```python
from build123d import *

# Parameters (mm, degrees)
SKETCH1_R           = 4.7
SKETCH1_R_2         = 2.5
BOSS_EXTRUDE1_DEPTH = 2.5
SKETCH2_R           = 4.7
BOSS_EXTRUDE2_DEPTH = 4.5
SKETCH3_R           = 1
CUT_EXTRUDE1_DEPTH  = 4.5
SKETCH6_W           = 6
SKETCH6_H           = 6
BOSS_EXTRUDE3_DEPTH = 8.31
SKETCH7_W           = 6
SKETCH7_H           = 6
BOSS_EXTRUDE4_DEPTH = 2
FILLET1_R           = 1
SKETCH8_R           = 1.75
CUT_EXTRUDE2_DEPTH  = 1.5
BOSS_EXTRUDE5_DEPTH = 0.5


with BuildPart() as part:
    # Sketch1 → Boss-Extrude1 (new body)
    with BuildSketch(Plane(origin=(0, 0, 0), x_dir=(1, 0, 0), z_dir=(0, 1, 0))):
        with Locations(Location((0, 0, 0), (0, 0, 270))):
            Circle(SKETCH1_R)
        with Locations(Location((0, 0, 0), (0, 0, 270))):
            Circle(SKETCH1_R_2, mode=Mode.SUBTRACT)
    extrude(amount=BOSS_EXTRUDE1_DEPTH)

    # Sketch2 → Boss-Extrude2 (add)
    with BuildSketch(Plane(origin=(0, 2.5, 0), x_dir=(1, 0, 0), z_dir=(0, 1, 0))):
        with Locations(Location((0, 0, 0), (0, 0, 270))):
            Circle(SKETCH2_R)
    extrude(amount=BOSS_EXTRUDE2_DEPTH)

    # Sketch3 → Cut-Extrude1 (cut)
    with BuildSketch(Plane(origin=(0, 7, 0), x_dir=(1, 0, 0), z_dir=(0, 1, 0))):
        with Locations(Location((0, 0, 0), (0, 0, 270))):
            Circle(SKETCH3_R)
    extrude(amount=-CUT_EXTRUDE1_DEPTH, mode=Mode.SUBTRACT)



with BuildPart() as body_2:
    # Sketch6 → Boss-Extrude3 (new body)
    with BuildSketch(Plane(origin=(4.7, 0, 0), x_dir=(0, 0, -1), z_dir=(1, 0, 0))):
        with Locations((0, 3.5)):
            Rectangle(SKETCH6_W, SKETCH6_H)
    extrude(amount=BOSS_EXTRUDE3_DEPTH)


with BuildPart() as part_1:
    add(part.part)

    add(body_2.part)  # Boss-Extrude4 merges body 2
    # Sketch7 → Boss-Extrude4 (add)
    with BuildSketch(Plane.ZY.offset(-4.7)):
        with Locations((0, 3.5)):
            Rectangle(SKETCH7_W, SKETCH7_H)
    extrude(amount=BOSS_EXTRUDE4_DEPTH)

    # Fillet1
    fillet1_edges = [part_1.edges().sort_by_distance(p)[0] for p in [
        (13.01, 3.5, -3),
        (13.01, 3.5, 3),
    ]]
    fillet(fillet1_edges, radius=FILLET1_R)

    # Sketch8 → Cut-Extrude2 (cut)
    with BuildSketch(Plane(origin=(13.01, 0, 0), x_dir=(0, 0, -1), z_dir=(1, 0, 0))):
        with Locations((0, 3.5)):
            Circle(SKETCH8_R)
    extrude(amount=-CUT_EXTRUDE2_DEPTH, mode=Mode.SUBTRACT)

    # Sketch9 → Boss-Extrude5 (add)
    with BuildSketch(Plane(origin=(0, 6.5, 0), x_dir=(1, 0, 0), z_dir=(0, 1, 0))):
        with BuildLine():
            Line((13.01, -2), (13.01, 2))
            ThreePointArc((13.01, 2), (12.717106781, 2.707106781), (12.01, 3))
            Line((12.01, 3), (3.618010503, 3))
            ThreePointArc((3.618010503, 3), (4.7, 0), (3.618010503, -3))
            Line((3.618010503, -3), (12.01, -3))
            ThreePointArc((12.01, -3), (12.717106781, -2.707106781), (13.01, -2))
        make_face()
    extrude(amount=BOSS_EXTRUDE5_DEPTH)


solid = part_1.part
```
The listing builds one solid part. Answer for the finished solid, in the listing's coordinates (mm). A direction names the side the tool comes from. Round coordinates to 2 decimals unless told otherwise and drop trailing zeros. Loops run counter-clockwise (first coordinate to the right, second up) from the corner with the lowest first, then second, coordinate; pieces in that order, holes last. Notation, with made-up numbers: (37.25, 89.25) -> (61.25, 89.25) arc R14 cw to (61.25, 101.25) -> close; hole circle Ø10 at (-3, 18.25). An arc over 180 degrees is marked (long way). Use one line per item in the form item = value.
1. The part is cut by section C-C on z = 0. Determine the outline of the cut face in (x, y).
Answer key:
outline = (-4.7, 0) -> (-2.5, 0) -> (-2.5, 2.5) -> (-1, 2.5) -> (-1, 7) -> (-4.7, 7) -> close; (1, 2.5) -> (2.5, 2.5) -> (2.5, 0) -> (4.7, 0) -> (4.7, 0.5) -> (13.01, 0.5) -> (13.01, 1.75) -> (11.51, 1.75) -> (11.51, 5.25) -> (13.01, 5.25) -> (13.01, 7) -> (1, 7) -> close
2. The part is cut by section D-D on y = 1.5. Determine the outline of the cut face in (x, z), and give its area (3 significant figures).
Answer key:
outline = (3.62, -3) -> (12.01, -3) arc R1 ccw to (13.01, -2) -> (13.01, 2) arc R1 ccw to (12.01, 3) -> (3.62, 3) arc R4.7 ccw (long way) to start; hole circle Ø5 at (0, 0)
area = 101 mm²
3. For a pull along Y with two mould halves and no side action, classify faces 1 (the cylindrical face through (-1, 5, 0)), 2 (the cylindrical face through (12.27, 1.79, 0.38)), 3 (the flat face through (-1, 2.5, 1)) as released by +Y, released by -Y, zero draft, split by the parting line, or undercut.
Answer key:
face_1 = zero draft
face_2 = undercut
face_3 = released by -Y
4. Find the intervals of material crossed by probe 1 along X at (y, z) = (4, 0); probe 2 along Z at (x, y) = (10, 3.25); probe 3 along Y at (x, z) = (11.9, 0), in increasing order. Write a range as [from, to].
Answer key:
probe_1 = [-4.7, -1], [1, 11.51]
probe_2 = [-3, 3]
probe_3 = [0.5, 1.75], [5.25, 7]
5. Flat-ended cylindrical pins translate along their axes: pin 1 Ø1.5 at (x, z) = (1, 1) entering from -Y; pin 2 Ø3 at (x, z) = (7.5, 1) entering from -Y; pin 3 Ø1.2 at (x, z) = (0, 0) entering from +Y; pin 4 Ø2 at (y, z) = (3.5, 0) entering from +X. Find the tip coordinate at first contact, or state that the pin passes through.
Answer key:
pin_1 = 2.5
pin_2 = 0.5
pin_3 = through
pin_4 = 11.51
6. The part is cut by section A-A on x = 0. Determine the outline of the cut face in (y, z), and give its area (3 significant figures).
Answer key:
outline = (0, -4.7) -> (7, -4.7) -> (7, -1) -> (2.5, -1) -> (2.5, -2.5) -> (0, -2.5) -> close; (0, 2.5) -> (2.5, 2.5) -> (2.5, 1) -> (7, 1) -> (7, 4.7) -> (0, 4.7) -> close
area = 44.3 mm²
7. A tool of negligible diameter and unlimited length cuts with its end or side. For faces 4 (the cylindrical face through (-2.44, 1.23, -0.54)), 5 (the flat face through (8, 4, -3)), 6 (the flat face through (8, 4, 3)), 7 (the flat face through (-2, 0, 2)), 8 (the flat face through (11.51, 4, 0)), from which of +Z, -Z, +X, -X, +Y, -Y can it reach the whole face along a straight path? Write none if from no direction.
Answer key:
face_4 = -Y
face_5 = -Z, +X, +Y, -Y
face_6 = +Z, +X, +Y, -Y
face_7 = +Z, -Z, +X, -X, -Y
face_8 = +X
8. The part is cut by section B-B on y = 5.5. Determine the outline of the cut face in (x, z).
Answer key:
outline = (3.62, -3) -> (12.01, -3) arc R1 ccw to (13.01, -2) -> (13.01, 2) arc R1 ccw to (12.01, 3) -> (3.62, 3) arc R4.7 ccw (long way) to start; hole circle Ø2 at (0, 0)
